Here's the drawing with two shaded views (mm, measured from the low corner). I have some questions. Coordinates: 2 decimals unless noted, no trailing zeros. Write each loop counter-clockwise with the first axis right and the second up, starting at its lowest first coordinate (ties: lowest second). Pieces come first, ordered by that corner, then holes. Notation, with made-up numbers: (31.25, 49) -> (49.25, 49) arc R25 cw to (49.25, 88) -> close; hole circle Ø5 at (31.25, 43.25). An arc over 180 degrees is marked (long way). Use one line per item in the form item = value.
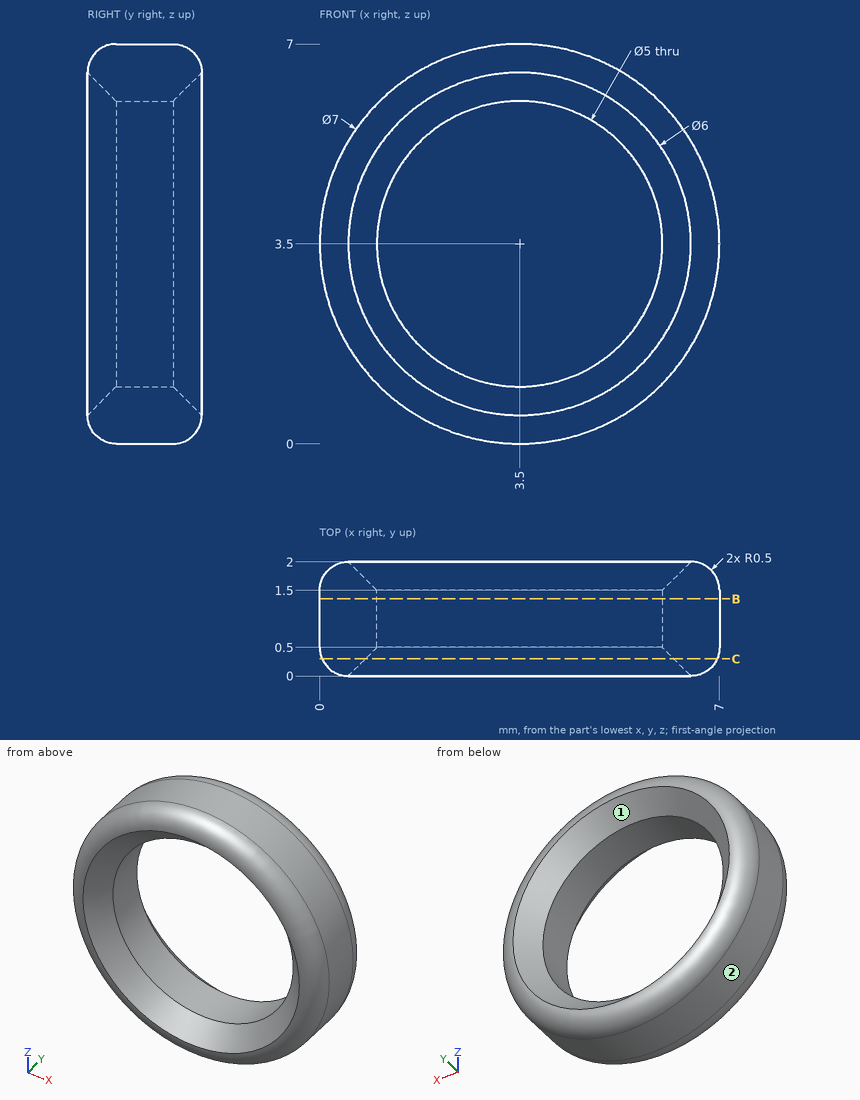
Q1. Will this pin go through, and if not, where does the flat tip stop? pin 1 (3 mm diameter, centred on x = 4.5, z = 4, fed in from -Y).
Return value:
pin_1 = 0.38
Q2. Thinking about a two-plate mould opening in X: for the marked faces 1 and 2, which applies, released by +X, released by -X, zero draft, split by the parting line, or undercut?
Return value:
face_1 = undercut
face_2 = split by the parting line
Q3. If I drill on line 1 (Z direction, x = 3.5, y = 1); line 2 (X direction, y = 1.3, z = 3); line 3 (Z direction, x = 5.5, y = 0.4), over which ranges is the centre line in solid material (lowest first)? Write a range as from..to.
Return value:
line_1 = 0..1, 6..7
line_2 = 0.04..1.05, 5.95..6.96
line_3 = 0.64..1.84, 5.16..6.36
Q4. Suppose I cut it at C-C (y = 0.3). Write out the boundary of the cut face in (x, z), then the cut area to 3 significant figures.
Return value:
outline = circle Ø6.92 at (3.5, 3.5); hole circle Ø5.4 at (3.5, 3.5)
area = 14.7 mm2
Q5. Suppose I cut it at B-B (y = 1.35). Write out the boundary of the cut face in (x, z).
Return value:
outline = circle Ø7 at (3.5, 3.5); hole circle Ø5 at (3.5, 3.5)
